Check sheet for the drawn part. Datum: minimum x, y, z corner. Units: mm. Round coordinates to 2 decimals unless told otherwise and drop trailing zeros. Write each loop counter-clockwise with the first axis right and the second up, starting at its lowest first coordinate (ties: lowest second). Pieces come first, ordered by that corner, then holes. Notation, with made-up numbers: (-13.5, 33.5) - (43.5, 33.5) arc R24 ccw to (43.5, 47.5) - close; hole circle Ø8 at (-33, 69). An arc over 180 degrees is marked (long way). Answer as a JSON object with one key per item and string values. Group by question number.
Item 1: Sectioned sample at C-C on x = 38.25. Record the boundary of the cut face in (y, z), plus the area to 3 significant figures.
Item 2: Sectioned sample at A-A on y = 105. Record the boundary of the cut face in (x, z), plus the area to 3 significant figures.
Item 3: Gauge pin test, flat ends, axial feed: P1, Ø3.5, axis at x = 81.75, y = 105, coming from the -Z side; P2, Ø1, axis at y = 77, z = 6.5, coming from the -X side (3 decimals); P3, Ø1.5, axis at y = 50, z = 2, coming from the -X side; P4, Ø1, axis at y = 46.5, z = 4, coming from the +X side. Record the tip position at first contact, or that the pin passes through.
Item 4: Sectioned sample at D-D on z = 3. Count the separate pieces of the cut face and the enclosed holes in it, plus the area to 3 significant figures.
Item 5: Thickness scan on line 1 (Y direction, x = 38.25, z = 2); line 2 (X direction, y = 5.5, z = 6.25); line 3 (Y direction, x = 47.5, z = 6.75). Record the ranges inside material, lowest first.
Item 6: Sectioned sample at B-B on y = 5. Record the boundary of the cut face in (x, z), plus the area to 3 significant figures.
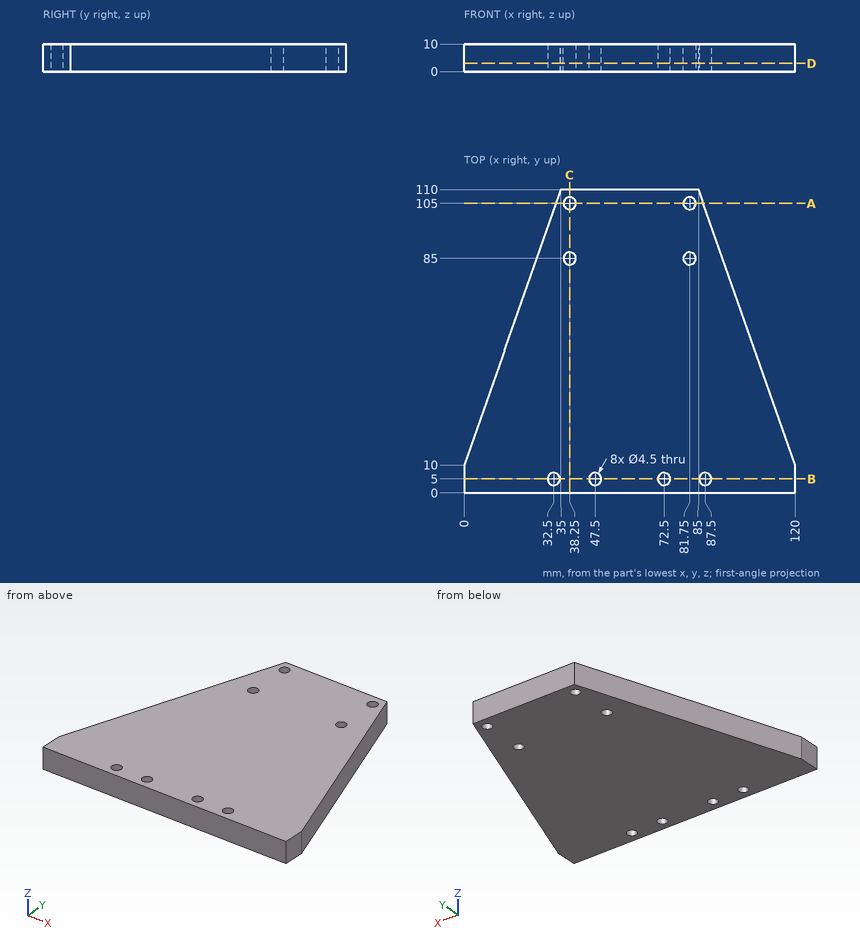
Completed:
{
 "1": {"outline": "(0, 0) - (82.75, 0) - (82.75, 10) - (0, 10) - close; (87.25, 0) - (102.75, 0) - (102.75, 10) - (87.25, 10) - close; (107.25, 0) - (110, 0) - (110, 10) - (107.25, 10) - close", "area": "1,010 mm²"},
 "2": {"outline": "(33.25, 0) - (36, 0) - (36, 10) - (33.25, 10) - close; (40.5, 0) - (79.5, 0) - (79.5, 10) - (40.5, 10) - close; (84, 0) - (86.75, 0) - (86.75, 10) - (84, 10) - close", "area": "445 mm²"},
 "3": {"P1": "through", "P2": "x = 23.275", "P3": "x = 13.74", "P4": "x = 107.4"},
 "4": {"separate pieces": "1", "enclosed holes": "8", "area": "9,570 mm²"},
 "5": {"line 1": "0 to 82.75, 87.25 to 102.75, 107.25 to 110", "line 2": "0 to 30.31, 34.69 to 45.31, 49.69 to 70.31, 74.69 to 85.31, 89.69 to 120", "line 3": "0 to 2.75, 7.25 to 110"},
 "6": {"outline": "(0, 0) - (30.25, 0) - (30.25, 10) - (0, 10) - close; (34.75, 0) - (45.25, 0) - (45.25, 10) - (34.75, 10) - close; (49.75, 0) - (70.25, 0) - (70.25, 10) - (49.75, 10) - close; (74.75, 0) - (85.25, 0) - (85.25, 10) - (74.75, 10) - close; (89.75, 0) - (120, 0) - (120, 10) - (89.75, 10) - close", "area": "1,020 mm²"}
}
